```python
from build123d import *

# Parameters (mm, degrees)
SKETCH085_R           = 1.8
EXTRUDE085_DEPTH      = 0.8
SKETCH083_W           = 82.8
SKETCH083_H           = 36
SKETCH083_R           = 1.8
EXTRUDE083_DEPTH      = 1.6
SKETCH080_R           = 2.25
EXTRUDE081_DEPTH      = 0.6
EXTRUDE081_DEPTH_BACK = 2.4
SKETCH081_R           = 3.4
EXTRUDE080_DEPTH      = 2.4
EXTRUDE079_DEPTH      = 1.2
SKETCH075_R           = 1.8
SKETCH075_R_2         = 2.8
SKETCH075_R_3         = 3
EXTRUDE078_DEPTH      = 2


with BuildPart() as extrude085:
    # Sketch085 → Extrude085 (new body)
    with BuildSketch(Plane.XZ):
        with BuildLine():
            ThreePointArc((-78.51, 31.3), (-76.035126, 32.325126), (-75.01, 34.8))
            Line((-75.01, 34.8), (-75.01, 39.2))
            Line((-82.8, 39.2), (-75.01, 39.2))
            Line((-82.8, 31.3), (-82.8, 39.2))
            Line((-82.8, 31.3), (-78.51, 31.3))
        make_face()
        with Locations((-78.51, 34.8)):
            Circle(SKETCH085_R, mode=Mode.SUBTRACT)
        with BuildLine():
            ThreePointArc((-9.1, 34.8), (-8.074874, 32.325126), (-5.6, 31.3))
            Line((-5.6, 31.3), (0, 31.3))
            Line((0, 39.2), (0, 31.3))
            Line((-9.1, 39.2), (0, 39.2))
            Line((-9.1, 39.2), (-9.1, 34.8))
        make_face()
        with Locations((-5.6, 34.8)):
            Circle(SKETCH085_R, mode=Mode.SUBTRACT)
        with BuildLine():
            ThreePointArc((-75.01, 7.6), (-76.035126, 10.074874), (-78.51, 11.1))
            Line((-82.8, 11.1), (-78.51, 11.1))
            Line((-82.8, 3.2), (-82.8, 11.1))
            Line((-75.01, 3.2), (-82.8, 3.2))
            Line((-75.01, 7.6), (-75.01, 3.2))
        make_face()
        with Locations((-78.51, 7.6)):
            Circle(SKETCH085_R, mode=Mode.SUBTRACT)
        with BuildLine():
            ThreePointArc((-5.6, 11.1), (-8.074874, 10.074874), (-9.1, 7.6))
            Line((-9.1, 7.6), (-9.1, 3.2))
            Line((-9.1, 3.2), (0, 3.2))
            Line((0, 3.2), (0, 11.1))
            Line((-5.6, 11.1), (0, 11.1))
        make_face()
        with Locations((-5.6, 7.6)):
            Circle(SKETCH085_R, mode=Mode.SUBTRACT)
    extrude(amount=EXTRUDE085_DEPTH)


with BuildPart() as extrude085_1:
    # Extrude085 placement: moved
    add(extrude085.part.moved(Location((0, -2.8, 0))))


with BuildPart() as cut048:
    # Sketch083 → Extrude083 (new body)
    with BuildSketch(Plane.XZ):
        with Locations((-41.4, 21.2)):
            Rectangle(SKETCH083_W, SKETCH083_H)
        with Locations((-78.51, 34.8)):
            Circle(SKETCH083_R, mode=Mode.SUBTRACT)
        with Locations((-5.6, 34.8)):
            Circle(SKETCH083_R, mode=Mode.SUBTRACT)
        with Locations((-5.6, 7.6)):
            Circle(SKETCH083_R, mode=Mode.SUBTRACT)
        with Locations((-78.51, 7.6)):
            Circle(SKETCH083_R, mode=Mode.SUBTRACT)
        with BuildLine():
            ThreePointArc((-65, 31.2), (-75, 21.2), (-65, 11.2))
            Line((-65, 11.2), (-19, 11.2))
            ThreePointArc((-19, 11.2), (-9, 21.2), (-19, 31.2))
            Line((-65, 31.2), (-19, 31.2))
        make_face(mode=Mode.SUBTRACT)
    extrude(amount=EXTRUDE083_DEPTH)


with BuildPart() as cut048_1:
    # Extrude083 placement: moved
    add(cut048.part.moved(Location((0, -2, 0))))

    # Cut048: cut Extrude085
    add(extrude085_1.part, mode=Mode.SUBTRACT)


with BuildPart() as extrude081:
    # Sketch080 → Extrude081 (new body, two sides)
    with BuildSketch(Plane.XZ) as extrude081_sk:
        with Locations((-18.6, 12.1)):
            Circle(SKETCH080_R)
        with Locations((-18.6, 30.3)):
            Circle(SKETCH080_R)
        with Locations((-43.2, 30.3)):
            Circle(SKETCH080_R)
        with Locations((-43.2, 12.1)):
            Circle(SKETCH080_R)
    extrude(amount=EXTRUDE081_DEPTH)
    extrude(extrude081_sk.sketch, amount=-EXTRUDE081_DEPTH_BACK)


with BuildPart() as extrude080:
    # Sketch081 → Extrude080 (new body)
    with BuildSketch(Plane.XZ):
        with Locations((-43.2, 30.3)):
            Circle(SKETCH081_R)
        with Locations((-18.6, 30.3)):
            Circle(SKETCH081_R)
        with Locations((-43.2, 12.1)):
            Circle(SKETCH081_R)
        with Locations((-18.6, 12.1)):
            Circle(SKETCH081_R)
    extrude(amount=-EXTRUDE080_DEPTH)


with BuildPart() as obj1:
    # Sketch077 → Extrude079 (new body)
    with BuildSketch(Plane.XZ):
        with BuildLine():
            Line((-27.2, 26.7), (-27.2, 15.7))
            ThreePointArc((-27.2, 15.7), (-24.2, 12.7), (-21.2, 15.7))
            Line((-21.2, 26.700018), (-21.2, 15.7))
            ThreePointArc((-21.2, 26.700018), (-24.200009, 29.7), (-27.2, 26.7))
        make_face()
    extrude(amount=EXTRUDE079_DEPTH)


with BuildPart() as fusion006:
    # Sketch075 → Extrude078 (new body)
    with BuildSketch(Plane.XZ):
        with BuildLine():
            Line((-82.8, 3.2), (0, 3.2))
            Line((0, 3.2), (0, 39.2))
            Line((-195.886839, 39.2), (0, 39.2))
            Line((-202.764796, 20.302968), (-195.886839, 39.2))
            ThreePointArc((-192.175575, -3.18451), (-192.085048, 10.987093), (-202.764796, 20.302968))
            Line((-192.175575, -3.18451), (-215.419579, -53.031439))
            ThreePointArc((-215.419579, -53.031439), (-218.578907, -66.677212), (-215.93199, -80.431568))
            Line((-215.93199, -80.431568), (-176.68528, -80.431568))
            Line((-147.645309, 8.944272), (-176.68528, -80.431568))
            ThreePointArc((-132.428405, 20), (-141.832969, 16.944272), (-147.645309, 8.944272))
            Line((-132.428405, 20), (-107.6, 20))
            ThreePointArc((-91.751972, 6.2), (-97.09286, 16.066483), (-107.6, 20))
            Line((-82.8, 6.2), (-91.751972, 6.2))
            Line((-82.8, 3.2), (-82.8, 6.2))
        make_face()
        with Locations((-213.443268, -76.831568)):
            Circle(SKETCH075_R, mode=Mode.SUBTRACT)
        with Locations((-179.304663, -76.831568)):
            Circle(SKETCH075_R, mode=Mode.SUBTRACT)
        with Locations((-184.079668, 34.8)):
            Circle(SKETCH075_R, mode=Mode.SUBTRACT)
        with Locations((-78.51, 34.8)):
            Circle(SKETCH075_R, mode=Mode.SUBTRACT)
        with Locations((-78.51, 7.6)):
            Circle(SKETCH075_R, mode=Mode.SUBTRACT)
        with Locations((-5.6, 34.8)):
            Circle(SKETCH075_R, mode=Mode.SUBTRACT)
        with Locations((-5.6, 7.6)):
            Circle(SKETCH075_R, mode=Mode.SUBTRACT)
        with Locations((-36.2, 21.2)):
            Circle(SKETCH075_R_2, mode=Mode.SUBTRACT)
        with Locations((-24.2, 26.7)):
            Circle(SKETCH075_R_3, mode=Mode.SUBTRACT)
        with Locations((-24.2, 15.7)):
            Circle(SKETCH075_R_3, mode=Mode.SUBTRACT)
        Polygon((-189.938695, 31.567195), (-192.332836, 24.989347), (-196.467483, 26.494236), (-194.073342, 33.072084), (-193.885404, 33.00368), (-190.126633, 31.635599), align=None, mode=Mode.SUBTRACT)
    extrude(amount=EXTRUDE078_DEPTH)

    # Cut045: cut obj1
    add(obj1.part, mode=Mode.SUBTRACT)

    # Fusion004: union Extrude080
    add(extrude080.part)

    # Cut046: cut Extrude081
    add(extrude081.part, mode=Mode.SUBTRACT)

    # Fusion006: union Cut048
    add(cut048_1.part)


solid = fusion006.part
```
Check sheet for the modelled part. Datum: model origin and axes. Units: mm. A direction names the side the tool comes from. Give positions to 0.01 mm unless a question says otherwise; leave off trailing zeros. Loops run counter-clockwise (first coordinate to the right, second up) from the corner with the lowest first, then second, coordinate; pieces in that order, holes last. Notation, with made-up numbers: M -39,71.25 L -13,71.25 A30 ccw -13,108.25 Z; hole C -1,-35 d3. An arc over 180 degrees is marked long. Answer as CSV lines item,"result".
Item 1: Scan lines: L1, parallel to Z at x = -18.6, y = 1.15; L2, parallel to Z at x = -24.2, y = -1.6; L3, parallel to Z at x = -78.51, y = -1. Record each from-to range of solid material in increasing order.
Reply:
L1,"8.7 to 9.85, 14.35 to 15.5, 26.9 to 28.05, 32.55 to 33.7"
L2,"3.2 to 12.7, 18.7 to 23.7, 29.7 to 39.2"
L3,"3.2 to 5.8, 9.4 to 33, 36.6 to 39.2"
Item 2: Sectioned sample at C-C, the plane z = -62. Enter the section's corners in (x, y).
Reply:
outline,"M -218.17,-2 L -170.7,-2 L -170.7,0 L -218.17,0 Z"
Item 3: Sectioned sample at A-A, the plane y = 1.05. Enter the section's corners in (x, z), then the cut area to 4 significant figures.
Reply:
outline,"C -43.2,12.1 d6.8; C -43.2,30.3 d6.8; C -18.6,12.1 d6.8; C -18.6,30.3 d6.8; hole C -43.2,12.1 d4.5; hole C -43.2,30.3 d4.5; hole C -18.6,12.1 d4.5; hole C -18.6,30.3 d4.5"
area,"81.65 mm^2"
Item 4: Draft check along X on faces 1 (the face through (-24, -1.2, 21)), 2 (the face through (-199.374, -0.986, 29.619)), 3 (the face through (-9, -3, 21)), 4 (the face through (-16, 2.4, 30)). Enter one of: pulls with the +X half, pulls with the -X half, needs draft (parallel to the pull), parting line crosses it, or undercut.
Reply:
face 1,"undercut"
face 2,"pulls with the -X half"
face 3,"undercut"
face 4,"needs draft"
Item 5: Sectioned sample at D-D, the plane x = -174.5. Enter the section's corners in (y, z), then the cut area to 3 significant figures.
Reply:
outline,"M -2,-73.71 L 0,-73.71 L 0,39.2 L -2,39.2 Z"
area,"226 mm^2"
Item 6: Sectioned sample at B-B, the plane x = -36.2. Enter the section's corners in (y, z).
Reply:
outline,"M -3.6,3.2 L 0,3.2 L 0,18.4 L -2,18.4 L -2,11.2 L -3.6,11.2 Z; M -3.6,31.2 L -2,31.2 L -2,24 L 0,24 L 0,39.2 L -3.6,39.2 Z"
Item 7: Depth check by flat-ended pin: pin 1 Ø0.8 at (x, y) = (-51.5, -3) entering from -Z; pin 2 Ø4 at (x, z) = (-4.5, 36) entering from -Y; pin 3 Ø1 at (x, y) = (-123, -0.5) entering from -Z; pin 4 Ø3 at (x, z) = (-179.3, -76.83) entering from +Y. Enter the tip coordinate at first touch or a pass-through.
Reply:
pin 1,"z = 3.2"
pin 2,"y = -2.8"
pin 3,"z = 20"
pin 4,"through"
Item 8: Set-up check for faces 5 (the face through (-42, 2.4, 10)), 6 (the face through (-81, -2.8, 35)), 7 (the face through (-42, -2, 21)), 8 (the face through (-141.719, -0.986, 17.026)), 9 (the face through (-40.06, 1.18, 10.8)): record each of +Z, -Z, +X, -X, +Y, -Y from which the full face is reachable in a straight line by a thin tool's end or side.
Reply:
face 5,"+Z, -Z, +X, -X, +Y"
face 6,"+Z, -X, -Y"
face 7,"-Y"
face 8,"-Z, +Y, -Y"
face 9,"+Y"
